Check sheet for the modelled part. Datum: model origin and axes. Units: mm. A direction names the side the tool comes from. Round coordinates to 2 decimals unless told otherwise and drop trailing zeros. Write each loop counter-clockwise with the first axis right and the second up, starting at its lowest first coordinate (ties: lowest second). Pieces come first, ordered by that corner, then holes.
from build123d import *

# Parameters (mm, degrees)
SKETCH1_R           = 18.5
BOSS_EXTRUDE1_DEPTH = 22.5
SKETCH2_R           = 1.6
CUT_EXTRUDE1_DEPTH  = 3.5
BOSS_EXTRUDE2_DEPTH = 21.3
BOSS_EXTRUDE3_DEPTH = 6.3
SKETCH4_R           = 14.5
BOSS_EXTRUDE4_DEPTH = 37.8
SKETCH5_R           = 5
BOSS_EXTRUDE5_DEPTH = 3
SKETCH6_R           = 1
BOSS_EXTRUDE6_DEPTH = 9
SKETCH7_W           = 0.5
SKETCH7_H           = 3
BOSS_EXTRUDE7_DEPTH = 6.5
CUT_EXTRUDE2_DEPTH  = 0.5
FILLET1_R           = 0.5


with BuildPart() as part:
    # Sketch1 → Boss-Extrude1 (new body)
    with BuildSketch(Plane.XY):
        with Locations(Location((0, 0, 0), (0, 0, 180))):
            Circle(SKETCH1_R)
    extrude(amount=BOSS_EXTRUDE1_DEPTH)

    # Sketch2 → Cut-Extrude1 (cut)
    with BuildSketch(Plane.XY.offset(22.5)):
        with Locations((-7.75, 13.423393759)):
            Circle(SKETCH2_R)
        with Locations((7.75, 13.423393759)):
            Circle(SKETCH2_R)
        with Locations((-15.5, 0)):
            Circle(SKETCH2_R)
        with Locations((-7.75, -13.423393759)):
            Circle(SKETCH2_R)
        with Locations((7.75, -13.423393759)):
            Circle(SKETCH2_R)
        with Locations((15.5, 0)):
            Circle(SKETCH2_R)
    extrude(amount=-CUT_EXTRUDE1_DEPTH, mode=Mode.SUBTRACT)

    # Sketch3 → Boss-Extrude2 (add)
    with BuildSketch(Plane.XY.offset(22.5)):
        with BuildLine():
            ThreePointArc((0, 9.5), (-2.5, 7), (0, 4.5))
            Line((0, 4.5), (0, 9.5))
        make_face()
        with BuildLine():
            Line((0, 9.5), (0, 4.5))
            ThreePointArc((0, 4.5), (1.767766953, 5.232233047), (2.5, 7))
            ThreePointArc((2.5, 7), (1.767766953, 8.767766953), (0, 9.5))
        make_face()
    extrude(amount=BOSS_EXTRUDE2_DEPTH)

    # Sketch3_3 → Boss-Extrude3 (add)
    with BuildSketch(Plane.XY.offset(22.5)):
        with BuildLine():
            ThreePointArc((0, 13), (-6, 7), (0, 1))
            Line((0, 1), (0, 4.5))
            ThreePointArc((0, 4.5), (-2.5, 7), (0, 9.5))
            Line((0, 9.5), (0, 13))
        make_face()
        with BuildLine():
            Line((0, 4.5), (0, 1))
            ThreePointArc((0, 1), (4.242640687, 2.757359313), (6, 7))
            ThreePointArc((6, 7), (4.242640687, 11.242640687), (0, 13))
            Line((0, 13), (0, 9.5))
            ThreePointArc((0, 9.5), (1.767766953, 8.767766953), (2.5, 7))
            ThreePointArc((2.5, 7), (1.767766953, 5.232233047), (0, 4.5))
        make_face()
    extrude(amount=BOSS_EXTRUDE3_DEPTH)

    # Sketch4 → Boss-Extrude4 (add)
    with BuildSketch(Plane(origin=(0, 0, 0), x_dir=(-1, 0, 0), z_dir=(0, 0, -1))):
        with Locations(Location((0, 0, 0), (0, 0, 180))):
            Circle(SKETCH4_R)
    extrude(amount=BOSS_EXTRUDE4_DEPTH)

    # Sketch5 → Boss-Extrude5 (add)
    with BuildSketch(Plane(origin=(0, 0, -37.8), x_dir=(-1, 0, 0), z_dir=(0, 0, -1))):
        Circle(SKETCH5_R)
    extrude(amount=BOSS_EXTRUDE5_DEPTH)

    # Sketch6 → Boss-Extrude6 (add)
    with BuildSketch(Plane(origin=(0, 0, -40.8), x_dir=(-1, 0, 0), z_dir=(0, 0, -1))):
        Circle(SKETCH6_R)
    extrude(amount=BOSS_EXTRUDE6_DEPTH)

    # Sketch7 → Boss-Extrude7 (add)
    with BuildSketch(Plane(origin=(0, 0, -37.8), x_dir=(-1, 0, 0), z_dir=(0, 0, -1))):
        with Locations((-11.75, 0)):
            Rectangle(SKETCH7_W, SKETCH7_H)
        with Locations((11.75, 0)):
            Rectangle(SKETCH7_W, SKETCH7_H)
    extrude(amount=BOSS_EXTRUDE7_DEPTH)

    # Sketch8 → Cut-Extrude2 (cut)
    with BuildSketch(Plane(origin=(12, 0, 0), x_dir=(0, 0, -1), z_dir=(1, 0, 0))):
        with BuildLine():
            Line((42.865122037, -0.320114275), (41.665122037, -0.320114275))
            ThreePointArc((41.665122037, -0.320114275), (41.345007763, 0), (41.665122037, 0.320114275))
            Line((41.665122037, 0.320114275), (42.865122037, 0.320114275))
            ThreePointArc((42.865122037, 0.320114275), (43.185236312, 0), (42.865122037, -0.320114275))
        make_face()
    cut_extrude2 = extrude(amount=-CUT_EXTRUDE2_DEPTH, mode=Mode.SUBTRACT)

    # Mirror2: Cut-Extrude2 across plane
    add(cut_extrude2.mirror(Plane(origin=(0, 0, 0), x_dir=(0, 0, 1), z_dir=(1, 0, 0))), mode=Mode.SUBTRACT)

    # Fillet1
    fillet1_edges = [part.edges().sort_by_distance(p)[0] for p in [
        (11.75, -1.5, -44.3),
        (11.75, 1.5, -44.3),
        (-11.75, 1.5, -44.3),
        (-11.75, -1.5, -44.3),
    ]]
    fillet(fillet1_edges, radius=FILLET1_R)

    # Chamfer1: read off the stored shape, not the designer's step
    # Chamfer1 outline → Chamfer1 (revolve, cut)
    with BuildSketch(Plane.XZ):
        Polygon((18.5, 22.5), (18.3, 22.5), (18.5, 22.3), align=None)
    revolve(axis=Axis((0, 0, 0), (0, 0, 1)), mode=Mode.SUBTRACT)

    # Chamfer1 2 outline → Chamfer1 2 (revolve, cut)
    with BuildSketch(Plane.XZ.offset(-7)):
        Polygon((6, 28.8), (5.8, 28.8), (6, 28.6), align=None)
        Polygon((2.3, 43.8), (2.5, 43.6), (2.5, 43.8), align=None)
    revolve(axis=Axis((0, 7, 0), (0, 0, 1)), mode=Mode.SUBTRACT)


solid = part.part
1. Sectioned sample at B-B, the plane z = -30. Enter the section's corners in (x, y).
2. Go/stop test with flat-tipped pins: pin 1 (3.5 mm diameter, centred on x = -7.75, y = 13.42, fed in from -Z); pin 2 (4 mm diameter, centred on y = 8.5, z = -39.5, fed in from -X); pin 3 (0.6 mm diameter, centred on x = 12, z = -42.5, fed in from +Y). Record where each tip stops, or that it passes through.
3. Release check for a two-part mould opening along Y. For faces 6 (the flat face through (0.1, 1.2, -40.8)), 7 (the flat face through (8, 13, 19)), 8 (the cylindrical face through (0, -1, -45)) record: released by +Y, released by -Y, zero draft, split by the parting line, or undercut.
4. Scan lines: line 1 along Y through (x, z) = (7.75, 21.65); line 2 along Z through (x, y) = (-6.5, 10.5); line 3 along Z through (x, y) = (3, -14.5). Record each from-to range of solid material in increasing order.
5. Sectioned sample at A-A, the plane z = 20. Enter the section's corners in (x, y), plus the area to 3 significant figures.
6. Set-up check for faces 1 (the flat face through (11, 10, 0)), 2 (the flat face through (12, 0, -41)), 3 (the cylindrical face through (-8.097, -14.985, 20.774)), 4 (the cylindrical face through (-8.54, 16.41, 10.99)), 5 (the flat face through (-12, 0, -41)): record each of +Z, -Z, +X, -X, +Y, -Y from which the full face is reachable in a straight line by a thin tool's end or side.
Computed values:
1. outline: circle Ø29 at (0, 0)
2. pin 1: stops at z = -37.8
2. pin 2: stops at x = -12.44
2. pin 3: stops at y = 1.5
3. face 6: zero draft
3. face 7: undercut
3. face 8: split by the parting line
4. line 1: y = -16.8 to -15.02, -11.82 to 11.82, 15.02 to 16.8
4. line 2: z = -37.8 to 22.5
4. line 3: z = 0 to 22.5
5. outline: circle Ø37 at (0, 0); hole circle Ø3.2 at (-15.5, 0); hole circle Ø3.2 at (-7.75, -13.42); hole circle Ø3.2 at (-7.75, 13.42); hole circle Ø3.2 at (7.75, -13.42); hole circle Ø3.2 at (7.75, 13.42); hole circle Ø3.2 at (15.5, 0)
5. area: 1,030 mm2
6. face 1: -Z
6. face 2: -Z, +X, +Y, -Y
6. face 3: +Z
6. face 4: +Z, -Z
6. face 5: -Z, -X, +Y, -Y
